```python
from build123d import *
from build123d.topology import SkipClean

# Parameters (mm, degrees)
SKETCH1_W               = 200
SKETCH1_H               = 150
BOSS_EXTRUDE1_DEPTH     = 25
CUT_EXTRUDE2_DEPTH      = 30
SHELL2_T                = -3
SKETCH6_R               = 2.5
CUT_EXTRUDE3_DEPTH      = 30
CUT_EXTRUDE4_DEPTH      = 30
CUT_EXTRUDE4_DEPTH_BACK = 30
SKETCH7_R               = 5
CHAMFER1_SIZE           = 5
SKETCH8_R               = 2.5
CUT_EXTRUDE5_DEPTH      = 10
SKETCH9_W               = 105
SKETCH9_H               = 150
CUT_EXTRUDE8_DEPTH      = 50
SKETCH10_R              = 2.5
CUT_EXTRUDE9_DEPTH      = 50
SKETCH11_W              = 20
SKETCH11_H              = 2.690986913
SKETCH11_W_2            = 20.020411306
SKETCH11_H_2            = 2.771183394
CUT_EXTRUDE10_DEPTH     = 28
SKETCH12_W              = 20
SKETCH12_H              = 3.926823093
CUT_EXTRUDE11_DEPTH     = 28
SKETCH_1_W              = 25
SKETCH_1_H              = 25
EXTRUDE_1_DEPTH         = 5
CHAMFER_1_SIZE          = 2
SKETCH_2_R              = 4
EXTRUDE_2_DEPTH         = 5
CHAMFER_4_SIZE          = 1


with BuildPart() as part:
    # Sketch1 → Boss-Extrude1 (new body)
    with BuildSketch(Plane.XY):
        Rectangle(SKETCH1_W, SKETCH1_H)
    extrude(amount=BOSS_EXTRUDE1_DEPTH)

    # Sketch5 → Cut-Extrude2 (cut)
    with BuildSketch(Plane(origin=(0, 0, 0), x_dir=(-1, 0, 0), z_dir=(0, 0, -1))):
        with BuildLine():
            Line((100, 75), (5, 75))
            ThreePointArc((5, 75), (24.038059223, 29.038059223), (70, 10))
            Line((70, 10), (100, 10))
            Line((100, 10), (100, 75))
        make_face()
        with BuildLine():
            ThreePointArc((70, -10), (24.038059223, -29.038059223), (5, -75))
            Line((5, -75), (100, -75))
            Line((100, -75), (100, -10))
            Line((100, -10), (70, -10))
        make_face()
        with BuildLine():
            Line((-80, -10), (-100, -10))
            Line((-100, -10), (-100, -75))
            Line((-100, -75), (-15, -75))
            ThreePointArc((-15, -75), (-34.038059223, -29.038059223), (-80, -10))
        make_face()
        with BuildLine():
            Line((-100, 75), (-100, 10))
            Line((-100, 10), (-80, 10))
            ThreePointArc((-80, 10), (-34.038059223, 29.038059223), (-15, 75))
            Line((-15, 75), (-100, 75))
        make_face()
    extrude(amount=-CUT_EXTRUDE2_DEPTH, mode=Mode.SUBTRACT)

    # Shell2
    shell2_openings = [part.faces().sort_by_distance(p)[0] for p in [
        (3.044348512, 0, 25),
    ]]
    offset(amount=SHELL2_T, openings=shell2_openings, kind=Kind.INTERSECTION)

    # Sketch6 → Cut-Extrude3 (cut)
    with BuildSketch(Plane(origin=(0, 0, 0), x_dir=(-1, 0, 0), z_dir=(0, 0, -1))):
        with Locations((-5, 65)):
            Circle(SKETCH6_R)
        with Locations((-5, -65)):
            Circle(SKETCH6_R)
    extrude(amount=-CUT_EXTRUDE3_DEPTH, mode=Mode.SUBTRACT)

    # Sketch7 → Cut-Extrude4 (cut, two sides: drawn at the far end of the back side and taken through both)
    with BuildSketch(Plane(origin=(0, 0, 0), x_dir=(1, 0, 0), z_dir=(0, 1, 0)).offset(-CUT_EXTRUDE4_DEPTH_BACK)):
        with Locations((-80, -25)):
            Circle(SKETCH7_R)
        with Locations((80, -25)):
            Circle(SKETCH7_R)
    extrude(amount=CUT_EXTRUDE4_DEPTH + CUT_EXTRUDE4_DEPTH_BACK, mode=Mode.SUBTRACT)

    # Chamfer1
    chamfer1_edges = [part.edges().sort_by_distance(p)[0] for p in [
        (-100, 0, 0),
        (5, 75, 0),
        (100, 0, 0),
        (5, -75, 0),
        (90, 10, 0),
        (34.038059223, 29.038059223, 0),
        (34.038059223, -29.038059223, 0),
        (90, -10, 0),
        (-24.038059223, -29.038059223, 0),
        (-85, -10, 0),
        (-24.038059223, 29.038059223, 0),
        (-85, 10, 0),
    ]]
    chamfer(chamfer1_edges, length=CHAMFER1_SIZE)

    # Sketch8 → Cut-Extrude5 (cut)
    with BuildSketch(Plane.XY.offset(3)):
        with Locations((-22, 15)):
            Circle(SKETCH8_R)
        with Locations((-22, -15)):
            Circle(SKETCH8_R)
    extrude(amount=-CUT_EXTRUDE5_DEPTH, mode=Mode.SUBTRACT)

    # Sketch9 → Cut-Extrude8 (cut)
    with BuildSketch(Plane.XY):
        with Locations((-47.5, 0)):
            Rectangle(SKETCH9_W, SKETCH9_H)
    extrude(amount=CUT_EXTRUDE8_DEPTH, mode=Mode.SUBTRACT)

    # Mirror4: part across plane


with BuildPart() as part_1:
    with SkipClean():  # the faces are left unmerged after this step: merging them gives an invalid solid
        add(part.part)
        add(part.part.mirror(Plane(origin=(5, 75, 50), x_dir=(0, 0, 1), z_dir=(-1, 0, 0))))

    # Sketch10 → Cut-Extrude9 (cut)
    with SkipClean():  # the faces are left unmerged after this step: merging them gives an invalid solid
        with BuildSketch(Plane.XY):
            with Locations((-14.7, 15)):
                Circle(SKETCH10_R)
            with Locations((-14.7, -15)):
                Circle(SKETCH10_R)
        extrude(amount=CUT_EXTRUDE9_DEPTH, mode=Mode.SUBTRACT)

    # Sketch11 → Cut-Extrude10 (cut)
    with SkipClean():  # the faces are left unmerged after this step: merging them gives an invalid solid
        with BuildSketch(Plane.ZY.offset(90)):
            with Locations((15, 11.345493457)):
                Rectangle(SKETCH11_W, SKETCH11_H)
            with Locations((15.010205653, -11.385591697)):
                Rectangle(SKETCH11_W_2, SKETCH11_H_2)
        extrude(amount=-CUT_EXTRUDE10_DEPTH, mode=Mode.SUBTRACT)

    # Sketch12 → Cut-Extrude11 (cut)
    with SkipClean():  # the faces are left unmerged after this step: merging them gives an invalid solid
        with BuildSketch(Plane(origin=(100, 0, 0), x_dir=(0, 0, -1), z_dir=(1, 0, 0))):
            with Locations((-15, 11.963411547)):
                Rectangle(SKETCH12_W, SKETCH12_H)
            with Locations((-15, -11.963411547)):
                Rectangle(SKETCH12_W, SKETCH12_H)
        extrude(amount=-CUT_EXTRUDE11_DEPTH, mode=Mode.SUBTRACT)

    # 草图1 → 凸台-拉伸1 (add)
    with SkipClean():  # the faces are left unmerged after this step: merging them gives an invalid solid
        with BuildSketch(Plane.XY.offset(3)):
            with Locations((12, 0.193209558)):
                Rectangle(SKETCH_1_W, SKETCH_1_H)
        extrude(amount=-EXTRUDE_1_DEPTH)

    # 倒角1
    chamfer_1_edges = [part_1.edges().sort_by_distance(p)[0] for p in [
        (12, 12.693209558, -2),
        (-0.5, 0.193209558, -2),
        (12, -12.306790442, -2),
        (24.5, 0.193209558, -2),
    ]]
    chamfer(chamfer_1_edges, length=CHAMFER_1_SIZE - 0.0001)  # a hair under: the kernel refuses the full size

    # 草图2 → 凸台-拉伸2 (add)
    with BuildSketch(Plane(origin=(0, 0, -2), x_dir=(-1, 0, 0), z_dir=(0, 0, -1))):
        with Locations(Location((-17, 5.693209558, 0), (0, 0, 180))):
            Circle(SKETCH_2_R)
        with Locations(Location((-7, 5.693209558, 0), (0, 0, 180))):
            Circle(SKETCH_2_R)
        with Locations(Location((-17, -5.306790442, 0), (0, 0, 180))):
            Circle(SKETCH_2_R)
        with Locations(Location((-7, -5.306790442, 0), (0, 0, 180))):
            Circle(SKETCH_2_R)
    extrude(amount=EXTRUDE_2_DEPTH)

    # 倒角4
    chamfer_4_edges = [part_1.edges().sort_by_distance(p)[0] for p in [
        (13, 5.693209558, -7),
        (13, -5.306790442, -7),
        (3, 5.693209558, -7),
        (3, -5.306790442, -7),
    ]]
    chamfer(chamfer_4_edges, length=CHAMFER_4_SIZE)


solid = part_1.part
```
Check sheet for the modelled part. Datum: model origin and axes. Units: mm. A direction names the side the tool comes from. Round coordinates to 2 decimals unless told otherwise and drop trailing zeros. Order: outer loops, then holes, each group sorted by start corner. A loop starts at its lowest first (then second) coordinate and runs counter-clockwise, first axis right, second up.
1) Section check B-B (x = -14.7). Give the number of separate pieces and of enclosed holes in the cut face, and give its area (3 significant figures).
2) Go/stop test with flat-tipped pins: pin 1 Ø13.5 at (x, z) = (-79.5, 11) entering from +Y; pin 2 Ø6.5 at (x, z) = (-65.5, 10) entering from -Y; pin 3 Ø10 at (x, z) = (27.5, 19.5) entering from +Y. Record where each tip stops, or that it passes through.
3) Tool access check on faces 1 (the flat face through (-78, -8, 3)), 2 (the flat face through (-88, 0, 3)), 3 (the flat face through (89, 7, 14)), 4 (the cylindrical face through (3.004, 5.517, -3.972)). Record the directions out of +Z, -Z, +X, -X, +Y, -Y that give a thin tool (end or side, any length) a straight path to the whole face; none if there is none.
4) Section check A-A (z = 8). Record the boundary of the cut face in (x, y).
5) Scan lines: line 1 (Y direction, x = -14, z = 1); line 2 (Y direction, x = -14.7, z = 1.6); line 3 (Z direction, x = -11, y = 24). Record each from-to range of solid material in increasing order.
6) Mould release check, pull along Y, two halves, no side actions. Record for faces 5 (the flat face through (-78, 8, 3)), 6 (the cylindrical face through (-16.7, 13.5, 1.5)), 7 (the flat face through (7, -5, -7)), 8 (the flat face through (97, 0, 14)): +Y half, -Y half, draft (parallel to the pull), parting line (faces both ways), or undercut.
Result:
1. separate pieces: 3
1. enclosed holes: 0
1. area: 408 mm2
2. pin 1: stops at y = 10
2. pin 2: stops at y = -10
2. pin 3: stops at y = 44.69
3. face 1: -Z, -X, -Y
3. face 2: -Z, -X, +Y, -Y
3. face 3: +Z
3. face 4: -Z
4. outline: (-90, -10) - (-62, -10) - (-62, -10.49) arc R65 cw to (-5, -75) - (15, -75) arc R65 cw to (72, -10.49) - (72, -10) - (100, -10) - (100, 10) - (72, 10) - (72, 10.49) arc R65 cw to (15, 75) - (-5, 75) arc R65 cw to (-62, 10.49) - (-62, 10) - (-90, 10) - close; hole (-87, -7) - (-70, -7) arc R68 cw to (-2.07, -72) - (12.07, -72) arc R68 cw to (80, -7) - (97, -7) - (97, 7) - (80, 7) arc R68 cw to (12.07, 72) - (-2.07, 72) arc R68 cw to (-70, 7) - (-87, 7) - close
5. line 1: y = -34.69 to -17.4, -12.6 to 12.6, 17.4 to 34.69
5. line 2: y = -34.74 to -17.5, -12.5 to 12.5, 17.5 to 34.74
5. line 3: z = 0 to 3
6. face 5: +Y half
6. face 6: undercut
6. face 7: draft
6. face 8: undercut
